Build history of the part. All positions in model axes, mm. A direction names the side the tool comes from. Give positions to 0.01 mm unless a question says otherwise; leave off trailing zeros. Order: outer loops, then holes, each group sorted by start corner. A loop starts at its lowest first (then second) coordinate and runs counter-clockwise, first axis right, second up. Notation, with made-up numbers: (-3.5, 68.25) - (29.5, 68.25) arc R15 cw to (29.5, 87.25) - close; hole circle Ø2 at (33, -14). An arc over 180 degrees is marked (long way). Write each question's results on one line, items separated by ' | '. Start each with the question number.
1) Cut at B-B on y = 19.5. List the corners of the cut face in (x, z), plus the area to 3 significant figures.
2) Drop flat-ended pins along their axis: pin 1 Ø7 at (x, y) = (2.5, 29) entering from +Z; pin 2 Ø7 at (x, y) = (22, 19) entering from +Z; pin 3 Ø15 at (y, z) = (28, 32.5) entering from -X. Give the stop position or say it passes through.
3) Drill centre lines: line 1 along X through (y, z) = (25.5, 3.5); line 2 along X through (y, z) = (3, 18.5); line 3 along Z through (x, y) = (36.5, 37.5). Where is each one in solid material? Low to high. Write a range as from..to.
4) Cut at C-C on x = 25.5. List the corners of the cut face in (y, z), plus the area to 3 significant figures.
5) Cut at A-A on z = 34.5. List the corners of the cut face in (x, y).
6) Cut at D-D on x = 17. List the corners of the cut face in (y, z).
7) Tool access for faces 5 (the face through (15, 20, 2)), 6 (the face through (36, 20, 25)), 7 (the face through (0, 20, 5)), 8 (the face through (27, 15, 35)), 9 (the face through (5, 20, 10)): list every direction of +Z, -Z, +X, -X, +Y, -Y with a clear straight run to the whole face (end or side of a thin tool).
8) Two-plate mould, pull along X, no slides. Class faces 1 (the face through (18, 15, 35)), 2 (the face through (9, 20, 25)), 3 (the face through (30, 20, 3)), 4 (the face through (41, 20, 10)): +X half, -X half, draft (parallel to the pull), parting line (faces both ways), or undercut.
from build123d import *

# Parameters (mm, degrees)
F0_W     = 9
F0_H     = 9
F1_DEPTH = 40
F2_DEPTH = 30


with BuildPart() as f1:
    # F0 (on Front) → F1 (new body)
    with BuildSketch(Plane.XZ):
        with Locations((22.5, 35.5)):
            Rectangle(F0_W, F0_H)
        Polygon((0, 10), (0, 0), (15, 0), (15, 5), (30, 5), (30, 0), (45, 0), (45, 10), (36, 10), (36, 40), (27, 40), (27, 31), (18, 31), (18, 40), (9, 40), (9, 10), align=None)
    extrude(amount=-F1_DEPTH)

    # F0 (on Front) → F2 (cut)
    with BuildSketch(Plane.XZ):
        with Locations((22.5, 35.5)):
            Rectangle(F0_W, F0_H)
    extrude(amount=-F2_DEPTH, mode=Mode.SUBTRACT)


solid = f1.part
Results:
1) outline: (0, 0) - (15, 0) - (15, 5) - (30, 5) - (30, 0) - (45, 0) - (45, 10) - (36, 10) - (36, 40) - (27, 40) - (27, 31) - (18, 31) - (18, 40) - (9, 40) - (9, 10) - (0, 10) - close | area: 1,100 mm^2
2) pin 1: z = 10 | pin 2: z = 31 | pin 3: x = 9
3) line 1: 0..15, 30..45 | line 2: 9..36 | line 3: 0..10
4) outline: (0, 5) - (40, 5) - (40, 40) - (30, 40) - (30, 31) - (0, 31) - close | area: 1,130 mm^2
5) outline: (9, 0) - (18, 0) - (18, 30) - (27, 30) - (27, 0) - (36, 0) - (36, 40) - (9, 40) - close
6) outline: (0, 5) - (40, 5) - (40, 40) - (0, 40) - close
7) face 5: -Z, +Y, -Y | face 6: +Z, +X, +Y, -Y | face 7: +Z, -Z, -X, +Y, -Y | face 8: +Z, -Y | face 9: +Z, -X, +Y, -Y
8) face 1: undercut | face 2: -X half | face 3: undercut | face 4: draft
